Autodesk Fusion 360 part; units mm, degrees
sketch "Skizze1" plane through (0, 0, 0) normal (0, 0, 1) x (1, 0, 0)
  line L0 (3.85, 0) -> (3.85, -10)
  line L1 (-3.85, -10) -> (-3.85, 0)
  arc A0 (-3.85, -10) -> (3.85, -10) centre (0, -10) ccw
  arc A1 (3.85, 0) -> (-3.85, 0) centre (0, 0) ccw
  circle A2 centre (0, 0) radius 1
  circle A3 centre (0, -10) radius 1
  dimension "d609" = 7.7
  dimension "d610" = 10
  dimension "d613" = 2
extrude "Extrusion1" add sketch "Skizze1" along normal blind 2
chamfer "Fase1" distance 0.5 angle 45 12 edges at (0, -13.85, 0) (3.85, -5, 0) (0, 3.85, 0) (-3.85, -5, 0) (-0.9323, -9.6384, 0) (-0.9323, 0.3616, 0) (-0.9323, 0.3616, 2) (-0.9323, -9.6384, 2) (0, -13.85, 2) (3.85, -5, 2) (0, 3.85, 2) (-3.85, -5, 2)
equation "d609 = 8 mm - 0.3 mm"
The model under review builds one solid part; all positions refer to its coordinate system, in mm. Give positions to 0.01 mm unless a question says otherwise; leave off trailing zeros. Write each loop counter-clockwise with the first axis right and the second up, starting at its lowest first coordinate (ties: lowest second). Pieces come first, ordered by that corner, then holes. Notation, with made-up numbers: (-27, 66) -> (16, 66) arc R11 cw to (16, 75) -> close; hole circle Ø11 at (-8.5, 76.5). An arc over 180 degrees is marked (long way). Answer in a Markdown table with one row per item.
1) Add section D-D on z = 1.75. State the section outline as (x, y) points, plus the area to 3 significant figures.
Worked answers:
| item | result |
|---|---|
| outline | (-3.6, -10) arc R3.6 ccw to (3.6, -10) -> (3.6, 0) arc R3.6 ccw to (-3.6, 0) -> close; hole circle Ø2.5 at (0, -10); hole circle Ø2.5 at (0, 0) |
| area | 103 mm² |
2) Add section C-C on y = -5.5. State the section outline as (x, z) points, plus the area to 3 significant figures.
Worked answers:
| item | result |
|---|---|
| outline | (-3.85, 0.5) -> (-3.35, 0) -> (3.35, 0) -> (3.85, 0.5) -> (3.85, 1.5) -> (3.35, 2) -> (-3.35, 2) -> (-3.85, 1.5) -> close |
| area | 14.9 mm² |
3) Mouldability with a two-part tool opening along X and no side actions: class faces 1 (the flat face through (0, -5, 2)), 2 (the cylindrical face through (0, 1, 1)), 3 (the conical face through (0.08, 3.49, 0.14)) as +X half, -X half, draft (parallel to the pull), parting line (faces both ways), or undercut.
Worked answers:
| item | result |
|---|---|
| face 1 | draft |
| face 2 | undercut |
| face 3 | parting line |
4) Add section A-A on x = 0. State the section outline as (y, z) points.
Worked answers:
| item | result |
|---|---|
| outline | (-13.85, 0.5) -> (-13.35, 0) -> (-11.5, 0) -> (-11, 0.5) -> (-11, 1.5) -> (-11.5, 2) -> (-13.35, 2) -> (-13.85, 1.5) -> close; (-9, 0.5) -> (-8.5, 0) -> (-1.5, 0) -> (-1, 0.5) -> (-1, 1.5) -> (-1.5, 2) -> (-8.5, 2) -> (-9, 1.5) -> close; (1, 0.5) -> (1.5, 0) -> (3.35, 0) -> (3.85, 0.5) -> (3.85, 1.5) -> (3.35, 2) -> (1.5, 2) -> (1, 1.5) -> close |
5) For L1, parallel to Y at x = 0, z = 1; L2, parallel to X at y = -10.25, z = 1.05; L3, parallel to X at y = 0.5, z = 1.3, list the stretches that pass through material, from the lowest coordinate up. Write a range as [from, to].
Worked answers:
| item | result |
|---|---|
| L1 | [-13.85, -11], [-9, -1], [1, 3.85] |
| L2 | [-3.84, -0.97], [0.97, 3.84] |
| L3 | [-3.82, -0.87], [0.87, 3.82] |
6) Add section B-B on z = 0.2. State the section outline as (x, y) points, plus the area to 4 significant figures.
Worked answers:
| item | result |
|---|---|
| outline | (-3.55, -10) arc R3.55 ccw to (3.55, -10) -> (3.55, 0) arc R3.55 ccw to (-3.55, 0) -> close; hole circle Ø2.6 at (0, -10); hole circle Ø2.6 at (0, 0) |
| area | 100.0 mm² |
7) Clearance check with flat-ended pins moving along their axes: P1, Ø1.5, axis at x = 0.5, y = 0.5, coming from the +Z side; P2, Ø2.5, axis at x = 0, y = -10, coming from the +Z side. State where each tip first meets the part, or that it passes through.
Worked answers:
| item | result |
|---|---|
| P1 | z = 1.96 |
| P2 | z = 1.75 |
